Answer from the drawing. Dimensions are ordinates in mm from the lowest x, y and z of the part. A direction names the side the tool comes from. Coordinates: 2 decimals unless noted, no trailing zeros. Order: outer loops, then holes, each group sorted by start corner. A loop starts at its lowest first (then second) coordinate and runs counter-clockwise, first axis right, second up.
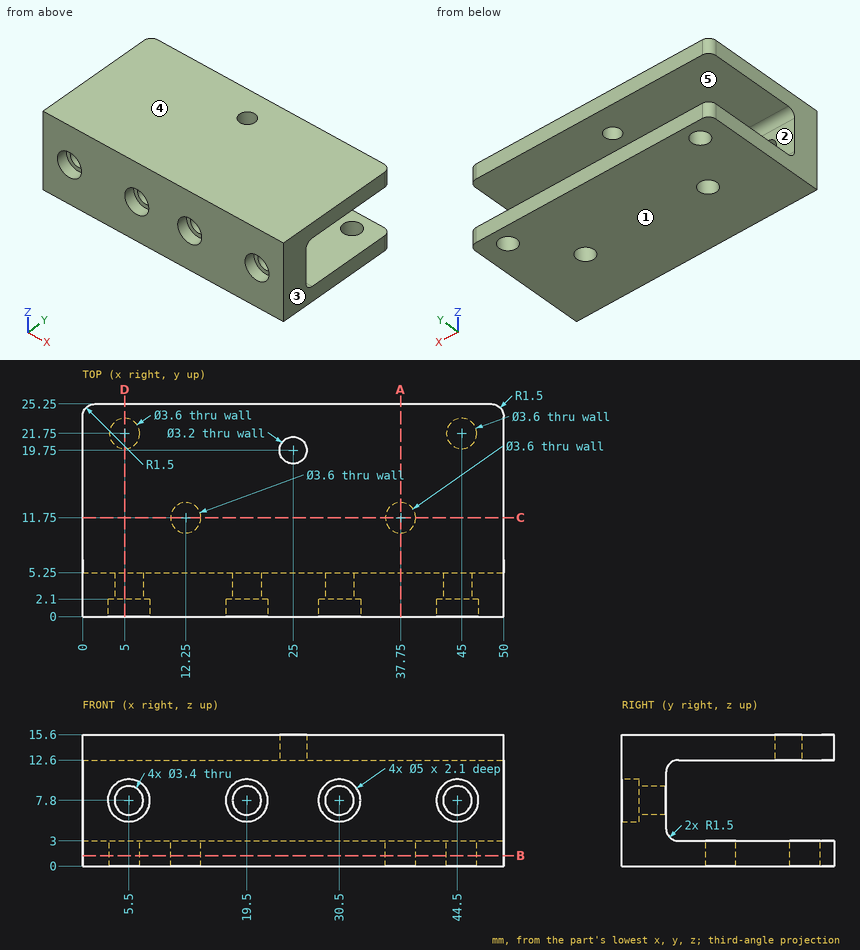
1) Section D-D (x = 5) is taken. Give the vertices of the cut face in (y, z).
2) Section C-C (y = 11.75) is taken. Give the vertices of the cut face in (x, z).
3) Section A-A (x = 37.75) is taken. Give the vertices of the cut face in (y, z), then the cut area to 3 significant figures.
4) Each of these flat-tipped pins is pushed along its axis until it touches: P1, Ø4, axis at x = 44.5, z = 7.8, coming from the -Y side; P2, Ø5, axis at x = 36.5, z = 6.5, coming from the -Y side; P3, Ø5.5, axis at x = 22.5, z = 6.5, coming from the +Y side; P4, Ø6.5, axis at x = 30.5, z = 7.8, coming from the +Y side. Where does it stop, or does it pass through?
5) Determine the mould class of the marked faces 3, 4 and 5 for opening direction Z: released by +Z, released by -Z, zero draft, split by the parting line, or undercut.
6) Section B-B (z = 1.25) is taken. Give the vertices of the cut face in (x, y).
7) Consider L1, parallel to X at y = 3.8, z = 7.8; L2, parallel to X at y = 1.4, z = 7.8; L3, parallel to Z at x = 3.5, y = 7.25. Determine where each line is inside the solid, lowest interval first.
8) A tool of negligible diameter and unlimited length cuts with its end or side. For the marked faces 1 and 2, from which of +Z, -Z, +X, -X, +Y, -Y can it reach the whole face along a straight path? Write none if from no direction.
Filled sheet:
1. outline: (0, 0) - (19.95, 0) - (19.95, 3) - (6.75, 3) arc R1.5 cw to (5.25, 4.5) - (5.25, 6.18) - (2.1, 6.18) - (2.1, 5.35) - (0, 5.35) - close; (0, 10.25) - (2.1, 10.25) - (2.1, 9.42) - (5.25, 9.42) - (5.25, 11.1) arc R1.5 cw to (6.75, 12.6) - (25.25, 12.6) - (25.25, 15.6) - (0, 15.6) - close; (23.55, 0) - (25.25, 0) - (25.25, 3) - (23.55, 3) - close
2. outline: (0, 0) - (10.45, 0) - (10.45, 3) - (0, 3) - close; (0, 12.6) - (50, 12.6) - (50, 15.6) - (0, 15.6) - close; (14.05, 0) - (35.95, 0) - (35.95, 3) - (14.05, 3) - close; (39.55, 0) - (50, 0) - (50, 3) - (39.55, 3) - close
3. outline: (0, 0) - (9.95, 0) - (9.95, 3) - (6.75, 3) arc R1.5 cw to (5.25, 4.5) - (5.25, 11.1) arc R1.5 cw to (6.75, 12.6) - (25.25, 12.6) - (25.25, 15.6) - (0, 15.6) - close; (13.55, 0) - (25.25, 0) - (25.25, 3) - (13.55, 3) - close
3. area: 192 mm2
4. P1: stops at y = 2.1
4. P2: stops at y = 0
4. P3: stops at y = 5.45
4. P4: stops at y = 5.25
5. face 3: zero draft
5. face 4: released by +Z
5. face 5: undercut
6. outline: (0, 0) - (50, 0) - (50, 23.75) arc R1.5 ccw to (48.5, 25.25) - (1.5, 25.25) arc R1.5 ccw to (0, 23.75) - close; hole circle Ø3.6 at (5, 21.75); hole circle Ø3.6 at (12.25, 11.75); hole circle Ø3.6 at (37.75, 11.75); hole circle Ø3.6 at (45, 21.75)
7. L1: x = 0 to 3.8, 7.2 to 17.8, 21.2 to 28.8, 32.2 to 42.8, 46.2 to 50
7. L2: x = 0 to 3, 8 to 17, 22 to 28, 33 to 42, 47 to 50
7. L3: z = 0 to 3, 12.6 to 15.6
8. face 1: -Z, +X, -X, +Y, -Y
8. face 2: +X, -X, +Y
